Part model, mm, in its own coordinate system. Coordinates: 2 decimals unless noted, no trailing zeros. Order: outer loops, then holes, each group sorted by start corner. A loop starts at its lowest first (then second) coordinate and runs counter-clockwise, first axis right, second up. Notation, with made-up numbers: (-32.5, 76) - (10.5, 76) arc R25 ccw to (10.5, 92) - close; hole circle Ø8 at (-9.75, 1.5). An arc over 180 degrees is marked (long way). Use a Markdown table: item, result. Add a question column.
1) Saw through at A-A on z = 0.95. Count the separate pieces of the cut face and the enclosed holes in it, then the cut area to 3 significant figures.
2) Wall check: L1, parallel to X at y = 64, z = 2.1; L2, parallel to Y at x = 30, z = 0.9; L3, parallel to X at y = 185.5, z = 0.4. Give the ranges that are in metal, low to high. Write a range as [from, to].
3) Saw through at B-B on x = 54.5. List the corners of the cut face in (y, z) (3 decimals).
```python
from build123d import *

# Parameters (mm, degrees)
SKETCH1_W                       = 120
SKETCH1_H                       = 234.78
BOSS_EXTRUDE1_DEPTH             = 3.175
CUT_EXTRUDE1_REACH              = 5.175
SKETCH2_W                       = 20
SKETCH2_H                       = 15
TAP_DRILL_FOR_M3X0_5_TAP1_D     = 3.4
TAP_DRILL_FOR_M3X0_5_TAP1_DEPTH = 3.18


with BuildPart() as part:
    # Sketch1 → Boss-Extrude1 (new body)
    with BuildSketch(Plane.XY):
        with Locations((60, 117.39)):
            Rectangle(SKETCH1_W, SKETCH1_H)
    extrude(amount=BOSS_EXTRUDE1_DEPTH)

    # Sketch2 → Cut-Extrude1 (cut, up to next)
    with BuildSketch(Plane.XY.offset(3.175), mode=Mode.PRIVATE) as cut_extrude1_sk1:
        with Locations((60, 227.28)):
            Rectangle(SKETCH2_W, SKETCH2_H)
    cut_extrude1_tool1 = extrude(cut_extrude1_sk1.sketch, amount=-CUT_EXTRUDE1_REACH, mode=Mode.PRIVATE) & part.part
    add(cut_extrude1_tool1.solids().sort_by_distance((60, 227.28, 3.175))[0], mode=Mode.SUBTRACT)

    # Tap Drill for M3x0.5 Tap1
    with Locations(Plane(origin=(42.952239605, 18.521605689, 3.175), x_dir=(-1, 0, 0), z_dir=(0, 0, 1))):
        with Locations((32.952239605, -210.31329226), (32.952239605, -165.478394311), (32.952239605, -105.478394311), (32.952239605, -75.478394311), (32.952239605, -45.478394311), (32.952239605, -15.478394311), (-67.047760395, -210.31329226), (32.952239605, -135.478394311), (12.952239605, 12.57670774), (-17.047760395, 12.57670774), (-47.047760395, 12.57670774), (-67.047760395, -165.478394311), (-67.047760395, -135.478394311), (-67.047760395, -105.478394311), (-67.047760395, -75.478394311), (-67.047760395, -45.478394311), (-67.047760395, -15.478394311)):
            Hole(TAP_DRILL_FOR_M3X0_5_TAP1_D / 2, depth=TAP_DRILL_FOR_M3X0_5_TAP1_DEPTH)


solid = part.part
```
Results are:
| question | item | result |
|---|---|---|
| 1 | separate pieces | 1 |
| 1 | enclosed holes | 17 |
| 1 | area | 27,700 mm2 |
| 2 | L1 | [0, 8.3], [11.7, 108.3], [111.7, 120] |
| 2 | L2 | [0, 4.24], [7.64, 234.78] |
| 2 | L3 | [0, 9.2], [10.8, 109.2], [110.8, 120] |
| 3 | outline | (0, 0) - (219.78, 0) - (219.78, 3.175) - (0, 3.175) - close |
